Autodesk Inventor part; units mm, degrees
ref_plane "o1_XY" through (0, -7.8105, 0) normal (1, 0, 0) x (0, 0, -1)
ref_plane "o1_YZ" through (0, -7.8105, 0) normal (0, 0, -1) x (0, 1, 0)
ref_plane "o1_ZX" through (0, -7.8105, 0) normal (0, 1, 0) x (1, 0, 0)
sketch "Sketch_5" plane through (0, 0, 0) normal (0, 0, 1) x (1, 0, 0)
  line L0 (69.85, 0) -> (-69.85, 0)
  line L1 (0, 6.9051) -> (0.263, 6.6421)
  line L2 (0.263, 6.6421) -> (0.635, 6.6421)
  line L3 (0.635, 6.6421) -> (1.27, 7.2771)
  line L4 (1.27, 7.2771) -> (68.58, 7.2771)
  line L5 (68.58, 7.2771) -> (69.215, 6.6421)
  line L6 (69.215, 6.6421) -> (69.587, 6.6421)
  line L7 (69.587, 6.6421) -> (69.85, 6.9051)
  line L8 (69.85, 6.9051) -> (68.9446, 7.8105)
  line L9 (68.9446, 7.8105) -> (0.9054, 7.8105)
  line L10 (0.9054, 7.8105) -> (0, 6.9051)
revolve "Revolution1" add sketch "Sketch_5" angle 360 about axis through (69.85, 0, 0) along (1, 0, 0)
ref_plane "o1_XY" through (0, -7.8105, 0) normal (1, 0, 0) x (0, 0, -1)
ref_plane "o1_YZ" through (0, -7.8105, 0) normal (0, 0, -1) x (0, 1, 0)
ref_plane "o1_ZX" through (0, -7.8105, 0) normal (0, 1, 0) x (1, 0, 0)
ref_plane "o2_XY" through (0, 7.8105, 0) normal (1, 0, 0) x (0, 0, -1)
ref_plane "o2_YZ" through (0, 7.8105, 0) normal (0, 0, -1) x (0, 1, 0)
ref_plane "o2_ZX" through (0, 7.8105, 0) normal (0, 1, 0) x (1, 0, 0)
ref_plane "t1_XY" through (34.925, 7.8105, 0) normal (1, 0, 0) x (0, 0, -1)
ref_plane "t1_YZ" through (34.925, 7.8105, 0) normal (0, 0, -1) x (0, 1, 0)
ref_plane "t1_ZX" through (34.925, 7.8105, 0) normal (0, 1, 0) x (1, 0, 0)
ref_plane "t2_XY" through (34.925, 0, -7.8105) normal (1, 0, 0) x (0, 0, -1)
ref_plane "t2_YZ" through (34.925, 0, -7.8105) normal (0, 0, -1) x (0, 1, 0)
ref_plane "t2_ZX" through (34.925, 0, -7.8105) normal (0, 1, 0) x (1, 0, 0)
ref_plane "t3_XY" through (34.925, -7.8105, 0) normal (1, 0, 0) x (0, 0, -1)
ref_plane "t3_YZ" through (34.925, -7.8105, 0) normal (0, 0, -1) x (0, 1, 0)
ref_plane "t3_ZX" through (34.925, -7.8105, 0) normal (0, 1, 0) x (1, 0, 0)
ref_plane "t4_XY" through (34.925, 0, 7.8105) normal (1, 0, 0) x (0, 0, -1)
ref_plane "t4_YZ" through (34.925, 0, 7.8105) normal (0, 0, -1) x (0, 1, 0)
ref_plane "t4_ZX" through (34.925, 0, 7.8105) normal (0, 1, 0) x (1, 0, 0)
ref_plane "tube1_XY" through (1.27, 0, 0) normal (1, 0, 0) x (0, 0, -1)
ref_plane "tube1_YZ" through (1.27, 0, 0) normal (0, 0, -1) x (0, 1, 0)
ref_plane "tube1_ZX" through (1.27, 0, 0) normal (0, 1, 0) x (1, 0, 0)
ref_plane "tube2_XY" through (68.58, 0, 0) normal (1, 0, 0) x (0, 0, -1)
ref_plane "tube2_YZ" through (68.58, 0, 0) normal (0, 0, -1) x (0, 1, 0)
ref_plane "tube2_ZX" through (68.58, 0, 0) normal (0, 1, 0) x (1, 0, 0)
properties part number "D-7516-2.75"
Work out the finished part from the listing and answer in its coordinate system (mm). A direction names the side the tool comes from. Coordinates: 2 decimals unless noted, no trailing zeros. Write each loop counter-clockwise with the first axis right and the second up, starting at its lowest first coordinate (ties: lowest second). Pieces come first, ordered by that corner, then holes. Notation, with made-up numbers: M 81,5.25 L 100,5.25 A22 ccw 100,15.25 Z; hole C 62,-5 d10. An arc over 180 degrees is marked long. Use one line per item in the form item = value. Start each with the question number.
1. Each of these flat-tipped pins is pushed along its axis until it touches: P1, Ø2, axis at x = 42, z = -5, coming from the +Y side; P2, Ø2, axis at x = 59.5, y = -3, coming from the -Z side; P3, Ø1, axis at x = 10, y = 1, coming from the +Z side. Where does it stop, or does it pass through?
2. The part is cut by section C-C (x = 60.5). Give the vertices of the cut face in (y, z), plus the area to 3 significant figures.
3. Straight lines are drawn through the part: probe 1 along Y at (x, z) = (54, 6.5); probe 2 along Z at (x, y) = (35.5, 5); probe 3 along Z at (x, y) = (69.35, 0). For each, find the intervals that lie inside material, in ascending order. Write a range as from..to.
4. A tool of negligible diameter and unlimited length cuts with its end or side. For faces 1 (the face through (69.404, -1.44, -6.484)), 2 (the face through (35.4, 6.94, 2.19)), from which of +Z, -Z, +X, -X, +Y, -Y can it reach the whole face along a straight path? Write none if from no direction.
5. The mould has two halves that part along Y. Classify faces 3 (the face through (34.449, -1.017, -7.744)), 4 (the face through (0.452, -1.44, -6.484)): released by +Y, released by -Y, zero draft, split by the parting line, or undercut.
Evaluation:
q1.P1 = 6.71
q1.P2 = -7.55
q1.P3 = 7.79
q2.outline = C 0,0 d15.62; hole C 0,0 d14.55
q2.area = 25.3 mm^2
q3.probe_1 = -4.33..-3.27, 3.27..4.33
q3.probe_2 = -6..-5.29, 5.29..6
q3.probe_3 = -7.41..-6.64, 6.64..7.41
q4.face_1 = +X, -X
q4.face_2 = none
q5.face_3 = split by the parting line
q5.face_4 = undercut
